```python
from build123d import *

# Parameters (mm, degrees)
SALIENTE_EXTRUIR1_DEPTH = 1
REDONDEO1_R             = 1
CROQUIS5_R              = 4
SALIENTE_EXTRUIR5_DEPTH = 0.6
CROQUIS2_R              = 1.98
CROQUIS2_R_2            = 1.18
SALIENTE_EXTRUIR2_DEPTH = 5


with BuildPart() as part:
    # Croquis1 → Saliente-Extruir1 (new body)
    with BuildSketch(Plane(origin=(0, 0, 0), x_dir=(1, 0, 0), z_dir=(0, 1, 0))):
        with BuildLine():
            Line((1.426584774, 9.845491503), (2.859425417, 5.435661447))
            ThreePointArc((2.859425417, 5.435661447), (3.404332313, 4.685661447), (4.286010191, 4.399186938))
            Line((4.286010191, 4.399186938), (8.922779911, 4.399186938))
            ThreePointArc((8.922779911, 4.399186938), (10.349364685, 3.36271243), (9.804457789, 1.685661447))
            Line((9.804457789, 1.685661447), (6.053232287, -1.039763413))
            ThreePointArc((6.053232287, -1.039763413), (5.508325391, -1.789763413), (5.508325391, -2.716814396))
            Line((5.508325391, -2.716814396), (6.941166033, -7.126644452))
            ThreePointArc((6.941166033, -7.126644452), (6.396259137, -8.803695435), (4.63290338, -8.803695435))
            Line((4.63290338, -8.803695435), (0.881677878, -6.078270576))
            ThreePointArc((0.881677878, -6.078270576), (0, -5.791796068), (-0.881677878, -6.078270576))
            Line((-0.881677878, -6.078270576), (-4.63290338, -8.803695435))
            ThreePointArc((-4.63290338, -8.803695435), (-6.396259137, -8.803695435), (-6.941166033, -7.126644452))
            Line((-6.941166033, -7.126644452), (-5.508325391, -2.716814396))
            ThreePointArc((-5.508325391, -2.716814396), (-5.508325391, -1.789763413), (-6.053232287, -1.039763413))
            Line((-6.053232287, -1.039763413), (-9.804457789, 1.685661447))
            ThreePointArc((-9.804457789, 1.685661447), (-10.349364685, 3.36271243), (-8.922779911, 4.399186938))
            Line((-8.922779911, 4.399186938), (-4.286010191, 4.399186938))
            ThreePointArc((-4.286010191, 4.399186938), (-3.404332313, 4.685661447), (-2.859425417, 5.435661447))
            Line((-2.859425417, 5.435661447), (-1.426584774, 9.845491503))
            ThreePointArc((-1.426584774, 9.845491503), (0, 10.881966011), (1.426584774, 9.845491503))
        make_face()
    extrude(amount=SALIENTE_EXTRUIR1_DEPTH)

    # Redondeo1
    redondeo1_edges = [part.edges().sort_by_distance(p)[0] for p in [
        (-6.224745712, 0, 4.921729424),
        (-6.396259137, 0, 8.803695435),
        (-2.757290629, 0, 7.440983006),
        (0, 0, 5.791796068),
        (2.757290629, 0, 7.440983006),
        (6.396259137, 0, 8.803695435),
        (6.224745712, 0, 4.921729424),
        (5.508325391, 0, 1.789763413),
        (7.928845038, 0, -0.322949017),
        (10.349364685, 0, -3.36271243),
        (6.604395051, 0, -4.399186938),
        (3.404332313, 0, -4.685661447),
        (2.143005096, 0, -7.640576475),
        (0, 0, -10.881966011),
        (-2.143005096, 0, -7.640576475),
        (-3.404332313, 0, -4.685661447),
        (-6.604395051, 0, -4.399186938),
        (-10.349364685, 0, -3.36271243),
        (-7.928845038, 0, -0.322949017),
        (-5.508325391, 0, 1.789763413),
    ]]
    fillet(redondeo1_edges, radius=REDONDEO1_R - 0.0001)  # a hair under: the kernel refuses the full size

    # Croquis5 → Saliente-Extruir5 (add)
    with BuildSketch(Plane(origin=(0, 1, 0), x_dir=(1, 0, 0), z_dir=(0, 1, 0))):
        with Locations(Location((0, 0, 0), (0, 0, 270))):
            Circle(CROQUIS5_R)
    extrude(amount=SALIENTE_EXTRUIR5_DEPTH)

    # Croquis2 → Saliente-Extruir2 (add)
    with BuildSketch(Plane(origin=(0, 1.6, 0), x_dir=(1, 0, 0), z_dir=(0, 1, 0))):
        with Locations(Location((0, 0, 0), (0, 0, 270))):
            Circle(CROQUIS2_R)
        with Locations(Location((0, 0, 0), (0, 0, 270))):
            Circle(CROQUIS2_R_2, mode=Mode.SUBTRACT)
    extrude(amount=SALIENTE_EXTRUIR2_DEPTH)


solid = part.part
```
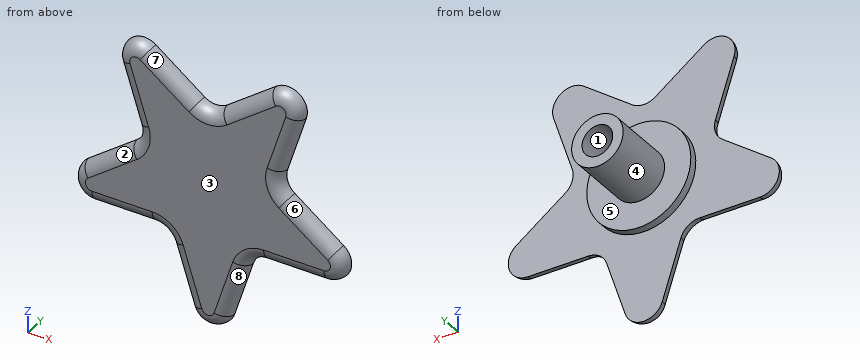
Check sheet for the modelled part. Datum: model origin and axes. Units: mm. Face numbers are marked on the shaded views. A direction names the side the tool comes from. Round coordinates to 2 decimals unless told otherwise and drop trailing zeros. Order: outer loops, then holes, each group sorted by start corner. A loop starts at its lowest first (then second) coordinate and runs counter-clockwise, first axis right, second up. Notation, with made-up numbers: (-4.75, 3.5) - (36.25, 3.5) arc R24 cw to (36.25, 17.5) - close; hole circle Ø2 at (87.5, -30.5). An arc over 180 degrees is marked (long way). Answer as CSV lines item,"result". Start each with the question number.
1) Section check A-A (y = 5.75). Record the cut outline in (x, z).
2) Scan lines: probe 1 along X at (y, z) = (2.85, 0); probe 2 along Y at (x, z) = (5.25, -3.25); probe 3 along Y at (x, z) = (-2.5, 0.5). Record each from-to range of solid material in increasing order.
3) Tool access check on the marked faces 5, 6, 7 and 8. Record the directions out of +Z, -Z, +X, -X, +Y, -Y that give a thin tool (end or side, any length) a straight path to the whole face; none if there is none.
4) Draft check along Z on the marked faces 1, 2, 3 and 4. Enter one of: +Z half, -Z half, draft (parallel to the pull), parting line (faces both ways), or undercut.
5) Depth check by flat-ended pin: pin 1 (0.7 mm diameter, centred on x = 0, z = 0.5, fed in from +Y). Enter the tip coordinate at first touch or a pass-through.
Determined:
1,outline,"circle Ø3.96 at (0, 0); hole circle Ø2.36 at (0, 0)"
2,probe 1,"-1.98 to -1.18, 1.18 to 1.98"
2,probe 2,"0 to 1"
2,probe 3,"0 to 1.6"
3,face 5,"+Y"
3,face 6,"+X, -Y"
3,face 7,"+Z, -Y"
3,face 8,"-Z, +X, -Y"
4,face 1,"undercut"
4,face 2,"undercut"
4,face 3,"draft"
4,face 4,"parting line"
5,pin 1,"y = 1.6"
